```python
from build123d import *

# Parameters (mm, degrees)
SKETCH1_R           = 20
BOSS_EXTRUDE1_DEPTH = 10
SCALE2_SCALE        = 0.1


with BuildPart() as part:
    # Sketch1 → Boss-Extrude1 (new body)
    with BuildSketch(Plane.XY):
        with BuildLine():
            Line((-25, -150), (-25, 150))
            ThreePointArc((-25, 150), (0, 175), (25, 150))
            Line((25, 150), (25, -150))
            ThreePointArc((25, -150), (0, -175), (-25, -150))
        make_face()
        with Locations((0, 150)):
            Circle(SKETCH1_R, mode=Mode.SUBTRACT)
        with Locations((0, -150)):
            Circle(SKETCH1_R, mode=Mode.SUBTRACT)
    extrude(amount=BOSS_EXTRUDE1_DEPTH)


with BuildPart() as part_1:
    # Scale2: scaled about (0, 0, 5)
    add(part.part.scale(SCALE2_SCALE).moved(Location((0, 0, 4.5))))


solid = part_1.part
```
Verification items for the finished model (mm, model axes). Round coordinates to 2 decimals unless told otherwise and drop trailing zeros. Order: outer loops, then holes, each group sorted by start corner. A loop starts at its lowest first (then second) coordinate and runs counter-clockwise, first axis right, second up. Notation, with made-up numbers: (-30, -34.75) -> (12, -34.75) arc R14 cw to (12, -28.75) -> close; hole circle Ø8 at (-26.75, 10). An arc over 180 degrees is marked (long way). Put each result on its own line as item: value. Start each with the question number.
(1) Material ranges on line 1 along Y through (x, z) = (0, 5.2); line 2 along X through (y, z) = (-15, 5); line 3 along Y through (x, z) = (-1.05, 5.4), recorded low to high.
(2) Depth check by flat-ended pin: pin 1 Ø2.5 at (x, y) = (0, -15) entering from -Z. Enter the tip coordinate at first touch or a pass-through.
(3) Section check A-A (x = 0). Enter the section's corners in (y, z).
(4) Draft check along X on faces 1 (the face through (0, 17, 5)), 2 (the face through (0.1, -17.5, 5)), 3 (the face through (2.5, 0, 5)). Enter one of: +X half, -X half, draft (parallel to the pull), parting line (faces both ways), or undercut.
(5) Section check C-C (x = -1.6). Enter the section's corners in (y, z).
(6) Section check B-B (z = 4.95). Enter the section's corners in (x, y), then the cut area to 3 significant figures.
Completed:
1. line 1: y = -17.5 to -17, -13 to 13, 17 to 17.5
1. line 2: x = -2.5 to -2, 2 to 2.5
1. line 3: y = -17.27 to -16.7, -13.3 to 13.3, 16.7 to 17.27
2. pin 1: passes through
3. outline: (-17.5, 4.5) -> (-17, 4.5) -> (-17, 5.5) -> (-17.5, 5.5) -> close; (-13, 4.5) -> (13, 4.5) -> (13, 5.5) -> (-13, 5.5) -> close; (17, 4.5) -> (17.5, 4.5) -> (17.5, 5.5) -> (17, 5.5) -> close
4. face 1: undercut
4. face 2: parting line
4. face 3: +X half
5. outline: (-16.92, 4.5) -> (-16.2, 4.5) -> (-16.2, 5.5) -> (-16.92, 5.5) -> close; (-13.8, 4.5) -> (13.8, 4.5) -> (13.8, 5.5) -> (-13.8, 5.5) -> close; (16.2, 4.5) -> (16.92, 4.5) -> (16.92, 5.5) -> (16.2, 5.5) -> close
6. outline: (-2.5, -15) arc R2.5 ccw to (2.5, -15) -> (2.5, 15) arc R2.5 ccw to (-2.5, 15) -> close; hole circle Ø4 at (0, -15); hole circle Ø4 at (0, 15)
6. area: 145 mm2
